The listing builds one solid part. Answer for the finished solid, in the listing's coordinates (mm). A direction names the side the tool comes from. Coordinates: 2 decimals unless noted, no trailing zeros. Write each loop counter-clockwise with the first axis right and the second up, starting at its lowest first coordinate (ties: lowest second). Pieces come first, ordered by that corner, then holes.
from build123d import *

# Parameters (mm, degrees)
SKETCH1_W                  = 12.7
SKETCH1_H                  = 22.606
BOSS_EXTRUDE1_DEPTH        = 3.175
SKETCH2_W                  = 12.7
SKETCH2_H                  = 3.175
BOSS_EXTRUDE2_DEPTH        = 6.604
SKETCH3_W                  = 12.7
SKETCH3_H                  = 22.606
BOSS_EXTRUDE3_DEPTH        = 3.175
SKETCH4_R                  = 3.4925
CUT_EXTRUDE1_DEPTH         = 13.954
SKETCH6_W                  = 3.175
SKETCH6_H                  = 12.954
BOSS_EXTRUDE4_DEPTH        = 3.175
SKETCH5_R                  = 1.7145
CUT_FOR_MOUNT_SCREWS_DEPTH = 23.606


with BuildPart() as part:
    # Sketch1 → Boss-Extrude1 (new body)
    with BuildSketch(Plane(origin=(0, 0, 0), x_dir=(1, 0, 0), z_dir=(0, 1, 0))):
        Rectangle(SKETCH1_W, SKETCH1_H)
    extrude(amount=BOSS_EXTRUDE1_DEPTH)

    # Sketch2 → Boss-Extrude2 (add)
    with BuildSketch(Plane(origin=(0, 3.175, 0), x_dir=(1, 0, 0), z_dir=(0, 1, 0))):
        with Locations((0, 9.7155)):
            Rectangle(SKETCH2_W, SKETCH2_H)
    extrude(amount=BOSS_EXTRUDE2_DEPTH)

    # Sketch3 → Boss-Extrude3 (add)
    with BuildSketch(Plane(origin=(0, 9.779, 0), x_dir=(1, 0, 0), z_dir=(0, 1, 0))):
        Rectangle(SKETCH3_W, SKETCH3_H)
    extrude(amount=BOSS_EXTRUDE3_DEPTH)

    # Sketch4 → Cut-Extrude1 (cut, through all)
    with BuildSketch(Plane(origin=(0, 12.954, 0), x_dir=(1, 0, 0), z_dir=(0, 1, 0))):
        with Locations((0, -4.953)):
            Circle(SKETCH4_R)
    extrude(amount=-CUT_EXTRUDE1_DEPTH, mode=Mode.SUBTRACT)

    # Sketch6 → Boss-Extrude4 (add)
    with BuildSketch(Plane(origin=(0, 0, -11.303), x_dir=(-1, 0, 0), z_dir=(0, 0, -1))):
        with Locations((-7.9375, 6.477)):
            Rectangle(SKETCH6_W, SKETCH6_H)
        with Locations((7.9375, 6.477)):
            Rectangle(SKETCH6_W, SKETCH6_H)
    extrude(amount=-BOSS_EXTRUDE4_DEPTH)

    # Sketch5 → cut for mount screws (cut, through all)
    with BuildSketch(Plane(origin=(0, 0, -11.303), x_dir=(-1, 0, 0), z_dir=(0, 0, -1))):
        with Locations((6.096, 6.477)):
            Circle(SKETCH5_R)
        with Locations((-6.096, 6.477)):
            Circle(SKETCH5_R)
    extrude(amount=-CUT_FOR_MOUNT_SCREWS_DEPTH, mode=Mode.SUBTRACT)


solid = part.part
Q1. Which of the six approach directions +Z, -Z, +X, -X, +Y, -Y give full straight-line access (tool end or side, diameter ignored) to faces 1 (the face through (-6.35, 11, 2)), 2 (the face through (0, 3.175, 1)), 3 (the face through (4.512, 5.82, -9.738)), 4 (the face through (0, 11, 11.303)), 5 (the face through (6.35, 11, 2))?
Answers below:
face 1: +Z, -X, +Y, -Y
face 2: +Z, +X, -X
face 3: +Z, -Z
face 4: +Z, +X, -X, +Y, -Y
face 5: +Z, +X, +Y, -Y
Q2. Find the intervals of material crossed by probe 1 along Z at (x, y) = (0, 11.05); probe 2 along Y at (x, z) = (-4.75, 8.5) (3 decimals); probe 3 along X at (y, z) = (6, -9.25) (3 decimals), in increasing order.
Answers below:
probe 1: z = -11.3 to 1.46, 8.45 to 11.3
probe 2: y = 0 to 3.175, 9.779 to 12.954
probe 3: x = -9.525 to -7.743, -4.449 to 4.449, 7.743 to 9.525
Q3. Determine the mould class of faces 6 (the face through (-0.76, 11.39, 8.36)), 7 (the face through (0, 2, 11.303)), 8 (the face through (0, 9.779, 1)) for opening direction Z: released by +Z, released by -Z, zero draft, split by the parting line, or undercut.
Answers below:
face 6: undercut
face 7: released by +Z
face 8: zero draft
Q4. Given pin 1 (2.5 mm diameter, centred on y = 2, z = -1, fed in from +X); pin 2 (5.5 mm diameter, centred on x = -6.096, y = 6.477, fed in from +Z); pin 3 (1.6 mm diameter, centred on y = 11, z = 1.5, fed in from -X), each flat-ended and moving along its own axis, determine where each tip first touches the part or whether it passes through.
Answers below:
pin 1: stops at x = 6.35
pin 2: stops at z = -8.13
pin 3: stops at x = -6.35
Q5. The part is cut by section D-D, the plane y = 5.75. Write down the section's boundary in (x, z) (3 decimals).
Answers below:
outline: (-9.525, -11.303) - (-7.649, -11.303) - (-7.649, -8.128) - (-9.525, -8.128) - close; (-4.543, -11.303) - (4.543, -11.303) - (4.543, -8.128) - (-4.543, -8.128) - close; (7.649, -11.303) - (9.525, -11.303) - (9.525, -8.128) - (7.649, -8.128) - close
Q6. The part is cut by section B-B, the plane z = -7.25. Write down the section's boundary in (x, y) (3 decimals), then the cut area to 3 significant figures.
Answers below:
outline: (-6.35, 0) - (6.35, 0) - (6.35, 3.175) - (-6.35, 3.175) - close; (-6.35, 9.779) - (6.35, 9.779) - (6.35, 12.954) - (-6.35, 12.954) - close
area: 80.6 mm2
Q7. The part is cut by section A-A, the plane x = 0. Write down the section's boundary in (y, z) (1 decimal), then the cut area to 3 significant figures.
Answers below:
outline: (0, -11.3) - (13, -11.3) - (13, 1.5) - (9.8, 1.5) - (9.8, -8.1) - (3.2, -8.1) - (3.2, 1.5) - (0, 1.5) - close; (0, 8.4) - (3.2, 8.4) - (3.2, 11.3) - (0, 11.3) - close; (9.8, 8.4) - (13, 8.4) - (13, 11.3) - (9.8, 11.3) - close
area: 120 mm2
Q8. The part is cut by section C-C, the plane x = -5.75. Write down the section's boundary in (y, z) (3 decimals), then the cut area to 3 significant figures.
Answers below:
outline: (0, -11.303) - (4.798, -11.303) - (4.798, -8.128) - (3.175, -8.128) - (3.175, 11.303) - (0, 11.303) - close; (8.156, -11.303) - (12.954, -11.303) - (12.954, 11.303) - (9.779, 11.303) - (9.779, -8.128) - (8.156, -8.128) - close
area: 154 mm2
